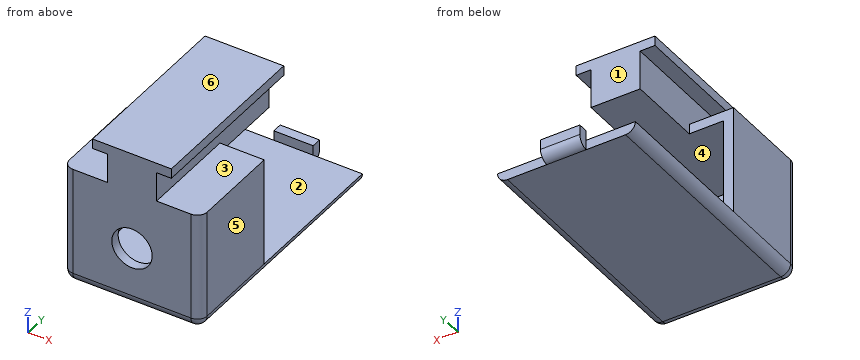
from build123d import *

# Parameters (mm, degrees)
F0_W      = 14
F0_H      = 25.5
F1_DEPTH  = 12
F2_T      = -1
F3_R      = 2.05
F4_DEPTH  = 25
F5_W      = 5
F5_H      = 10
F6_DEPTH  = 3
F7_R      = 1
F8_W      = 5
F8_H      = 3
F9_DEPTH  = 7.75
F10_W     = 8
F10_H     = 17.75
F11_DEPTH = 1
F13_DEPTH = 11
F14_W     = 4
F14_H     = 2
F15_DEPTH = 1
F16_R     = 1


with BuildPart() as f1:
    # F0 (on Top) → F1 (new body)
    with BuildSketch(Plane.XY):
        Rectangle(F0_W, F0_H)
    extrude(amount=F1_DEPTH)

    # F2
    f2_openings = [f1.faces().sort_by_distance(p)[0] for p in [
        (0, 12.75, 6),
    ]]
    offset(amount=F2_T, openings=f2_openings)

    # F3 (on face) → F4 (cut)
    with BuildSketch(Plane.XZ.offset(12.75)):
        with Locations((0, 6)):
            Circle(F3_R)
    extrude(amount=-F4_DEPTH, mode=Mode.SUBTRACT)

    # F5 (on face) → F6 (join)
    with BuildSketch(Plane.XY.offset(12)):
        Rectangle(F5_W, F5_H)
    extrude(amount=F6_DEPTH)

    # F7
    f7_edges = [f1.edges().sort_by_distance(p)[0] for p in [
        (7, 0, 0),
        (-7, 0, 0),
        (-7, -12.75, 6),
        (0, -12.75, 0),
        (7, -12.75, 6),
    ]]
    fillet(f7_edges, radius=F7_R)

    # F8 (on face) → F9 (join)
    with BuildSketch(Plane.XZ.offset(5)):
        with Locations((0, 13.5)):
            Rectangle(F8_W, F8_H)
    extrude(amount=F9_DEPTH)

    # F10 (on face) → F11 (join)
    with BuildSketch(Plane.XY.offset(15)):
        with Locations((0, -3.875)):
            Rectangle(F10_W, F10_H)
    extrude(amount=F11_DEPTH)

    # F12 (on face) → F13 (cut)
    with BuildSketch(Plane.XY.offset(12)):
        Polygon((7, -2.75), (7, 12.75), (-7, 12.75), (-7, -2.75), (-2.5, -2.75), (-2.5, 5), (2.5, 5), (2.5, -2.75), align=None)
    extrude(amount=-F13_DEPTH, mode=Mode.SUBTRACT)

    # F14 (on face) → F15 (join)
    with BuildSketch(Plane(origin=(0, 12.75, 0), x_dir=(-1, 0, 0), z_dir=(0, 1, 0))):
        with Locations((0, 1)):
            Rectangle(F14_W, F14_H)
    extrude(amount=F15_DEPTH)

    # F16
    f16_edges = [f1.edges().sort_by_distance(p)[0] for p in [
        (0, 13.75, 0),
    ]]
    fillet(f16_edges, radius=F16_R)


solid = f1.part
Can you work these out from the model? Positions are in its coordinate system, mm. Face numbers are marked on the shaded views. A direction names the side the tool comes from. Coordinates: 2 decimals unless noted, no trailing zeros. Write each loop counter-clockwise with the first axis right and the second up, starting at its lowest first coordinate (ties: lowest second). Pieces come first, ordered by that corner, then holes.
Q1. Imagine slicing it at D-D, the plane z = 9.75. List the corners of the cut face in (x, y) for me.
Results found:
outline: (-7, -11.75) arc R1 ccw to (-6, -12.75) - (6, -12.75) arc R1 ccw to (7, -11.75) - (7, -2.75) - (6, -2.75) - (6, -11.75) - (-6, -11.75) - (-6, -2.75) - (-7, -2.75) - close
Q2. Which directions (+Z, -Z, +X, -X, +Y, -Y) give clear straight access to the entire face, cutting with the end or side of a thin tool? Please do the marked faces 1, 2 and 3.
Results found:
face 1: +Z, +X, -X, +Y
face 2: none
face 3: +X, +Y, -Y
Q3. If we mould it in two halves opening along X, with no side actions, what happens to the marked faces 4, 5 and 6? For each: +X half, -X half, draft (parallel to the pull), parting line (faces both ways), or undercut.
Results found:
face 4: undercut
face 5: +X half
face 6: draft
Q4. Imagine slicing it at A-A, the plane z = 6. List the corners of the cut face in (x, y) for me.
Results found:
outline: (-7, -11.75) arc R1 ccw to (-6, -12.75) - (-2.05, -12.75) - (-2.05, -11.75) - (-6, -11.75) - (-6, -2.75) - (-7, -2.75) - close; (2.05, -12.75) - (6, -12.75) arc R1 ccw to (7, -11.75) - (7, -2.75) - (6, -2.75) - (6, -11.75) - (2.05, -11.75) - close
Q5. Imagine slicing it at B-B, the plane x = 0. List the corners of the cut face in (y, z) for me.
Results found:
outline: (-12.75, 1) arc R1 ccw to (-11.75, 0) - (12.75, 0) arc R1 ccw to (13.75, 1) - (13.75, 2) - (12.75, 2) - (12.75, 1) - (-11.75, 1) - (-11.75, 3.95) - (-12.75, 3.95) - close; (-12.75, 8.05) - (-11.75, 8.05) - (-11.75, 11) - (5, 11) - (5, 16) - (-12.75, 16) - close
Q6. For P1, Ø0.8, axis at x = -0.5, y = 13.5, coming from the +Z side; P2, Ø0.8, axis at x = 4, z = 0.5, coming from the +Y side; P3, Ø3.5, axis at x = 4.5, z = 5.5, coming from the +Y side, each with a flat end and sliding along its axis, tell me the tip position at first contact or that it passes through.
Results found:
P1: stops at z = 2
P2: stops at y = 12.75
P3: stops at y = -2.75
Q7. Please list where these lines run through material, in increasing order: L1, parallel to Z at x = 3.5, y = -10.5; L2, parallel to X at y = -11, z = 4.75; L3, parallel to Z at x = -1.75, y = -5.
Results found:
L1: z = 0 to 1, 11 to 12, 15 to 16
L2: x = -7 to -6, 6 to 7
L3: z = 0 to 1, 11 to 16
Q8. Imagine slicing it at C-C, the plane y = -3.75. List the corners of the cut face in (x, z) for me.
Results found:
outline: (-7, 1) arc R1 ccw to (-6, 0) - (6, 0) arc R1 ccw to (7, 1) - (7, 12) - (2.5, 12) - (2.5, 15) - (4, 15) - (4, 16) - (-4, 16) - (-4, 15) - (-2.5, 15) - (-2.5, 12) - (-7, 12) - close; hole (-6, 1) - (6, 1) - (6, 11) - (-6, 11) - close
